```python
from build123d import *

# Parameters (mm, degrees)
SKETCH1_W                                      = 27.99999988
SKETCH1_H                                      = 28
BOSS_EXTRUDE1_DEPTH                            = 4.7625
SKETCH2_R                                      = 12.065
CUT_EXTRUDE1_DEPTH                             = 2.286
SKETCH3_R                                      = 9.652
CUT_EXTRUDE2_DEPTH                             = 3.4765
CSK_FOR_2_FLAT_HEAD_MACHINE_SCREW1_D           = 2.4384
CSK_FOR_2_FLAT_HEAD_MACHINE_SCREW1_CSINK_D     = 4.3688
CSK_FOR_2_FLAT_HEAD_MACHINE_SCREW1_CSINK_ANGLE = 82


with BuildPart() as part:
    # Sketch1 → Boss-Extrude1 (new body)
    with BuildSketch(Plane.XY):
        Rectangle(SKETCH1_W, SKETCH1_H)
    extrude(amount=BOSS_EXTRUDE1_DEPTH)

    # Sketch2 → Cut-Extrude1 (cut)
    with BuildSketch(Plane.XY.offset(4.7625)):
        Circle(SKETCH2_R)
    extrude(amount=-CUT_EXTRUDE1_DEPTH, mode=Mode.SUBTRACT)

    # Sketch3 → Cut-Extrude2 (cut, through all)
    with BuildSketch(Plane.XY.offset(2.4765)):
        Circle(SKETCH3_R)
    extrude(amount=-CUT_EXTRUDE2_DEPTH, mode=Mode.SUBTRACT)

    # CSK for #2 Flat Head Machine Screw1 (through all)
    with Locations(Plane(origin=(0, 0, 0), x_dir=(-1, 0, 0), z_dir=(0, 0, -1))):
        with Locations((11.61874994, 11.61875), (11.61874994, -11.61875), (-11.61874994, -11.61875), (-11.61874994, 11.61875)):
            CounterSinkHole(CSK_FOR_2_FLAT_HEAD_MACHINE_SCREW1_D / 2, CSK_FOR_2_FLAT_HEAD_MACHINE_SCREW1_CSINK_D / 2, counter_sink_angle=CSK_FOR_2_FLAT_HEAD_MACHINE_SCREW1_CSINK_ANGLE)


solid = part.part
```
Geometry check sheet. Reference: the model listing, model coordinates, mm. A direction names the side the tool comes from. Give positions to 0.01 mm unless a question says otherwise; leave off trailing zeros. Order: outer loops, then holes, each group sorted by start corner. A loop starts at its lowest first (then second) coordinate and runs counter-clockwise, first axis right, second up.
1. Section check D-D, the plane z = 4.35. Enter the section's corners in (x, y) (3 decimals), and give its area (3 significant figures).
2. Section check C-C, the plane z = 1.8. Enter the section's corners in (x, y).
3. Release check for a two-part mould opening along X. For faces 1 (the face through (10.65, 10.88, 2.96)), 2 (the face through (-14, 0, 2)), 3 (the face through (-10, 3, 0)) record: pulls with the +X half, pulls with the -X half, needs draft (parallel to the pull), parting line crosses it, or undercut.
4. Gauge pin test, flat ends, axial feed: pin 1 Ø7 at (x, y) = (0, -4.5) entering from +Z (3 decimals); pin 2 Ø4 at (x, y) = (-11.62, -11.62) entering from -Z. Record the tip position at first contact, or that the pin passes through.
5. Thickness scan on L1, parallel to Y at x = 0, z = 1; L2, parallel to Y at x = 11, z = 1.35; L3, parallel to Z at x = -2.25, y = -11.5. Record the ranges inside material, lowest first.
6. Access from +Z, -Z, +X, -X, +Y, -Y to the whole of each face (thin tool, end or side, straight path). Record for faces 4 (the face through (10.72, -10.795, 2.962)), 5 (the face through (4, 9, 2.476)).
7. Section check A-A, the plane x = 0. Enter the section's corners in (y, z) (1 decimal).
Values follow:
1. outline: (-14, -14) - (14, -14) - (14, 14) - (-14, 14) - close; hole circle Ø2.438 at (-11.619, -11.619); hole circle Ø2.438 at (-11.619, 11.619); hole circle Ø24.13 at (0, 0); hole circle Ø2.438 at (11.619, -11.619); hole circle Ø2.438 at (11.619, 11.619)
1. area: 308 mm2
2. outline: (-14, -14) - (14, -14) - (14, 14) - (-14, 14) - close; hole circle Ø2.44 at (-11.62, -11.62); hole circle Ø2.44 at (-11.62, 11.62); hole circle Ø19.3 at (0, 0); hole circle Ø2.44 at (11.62, -11.62); hole circle Ø2.44 at (11.62, 11.62)
3. face 1: undercut
3. face 2: pulls with the -X half
3. face 3: needs draft
4. pin 1: passes through
4. pin 2: stops at z = 0.21
5. L1: y = -14 to -9.65, 9.65 to 14
5. L2: y = -14 to -12.67, -10.57 to 10.57, 12.67 to 14
5. L3: z = 0 to 2.48
6. face 4: +Z, -Z
6. face 5: +Z
7. outline: (-14, 0) - (-9.7, 0) - (-9.7, 2.5) - (-12.1, 2.5) - (-12.1, 4.8) - (-14, 4.8) - close; (9.7, 0) - (14, 0) - (14, 4.8) - (12.1, 4.8) - (12.1, 2.5) - (9.7, 2.5) - close
